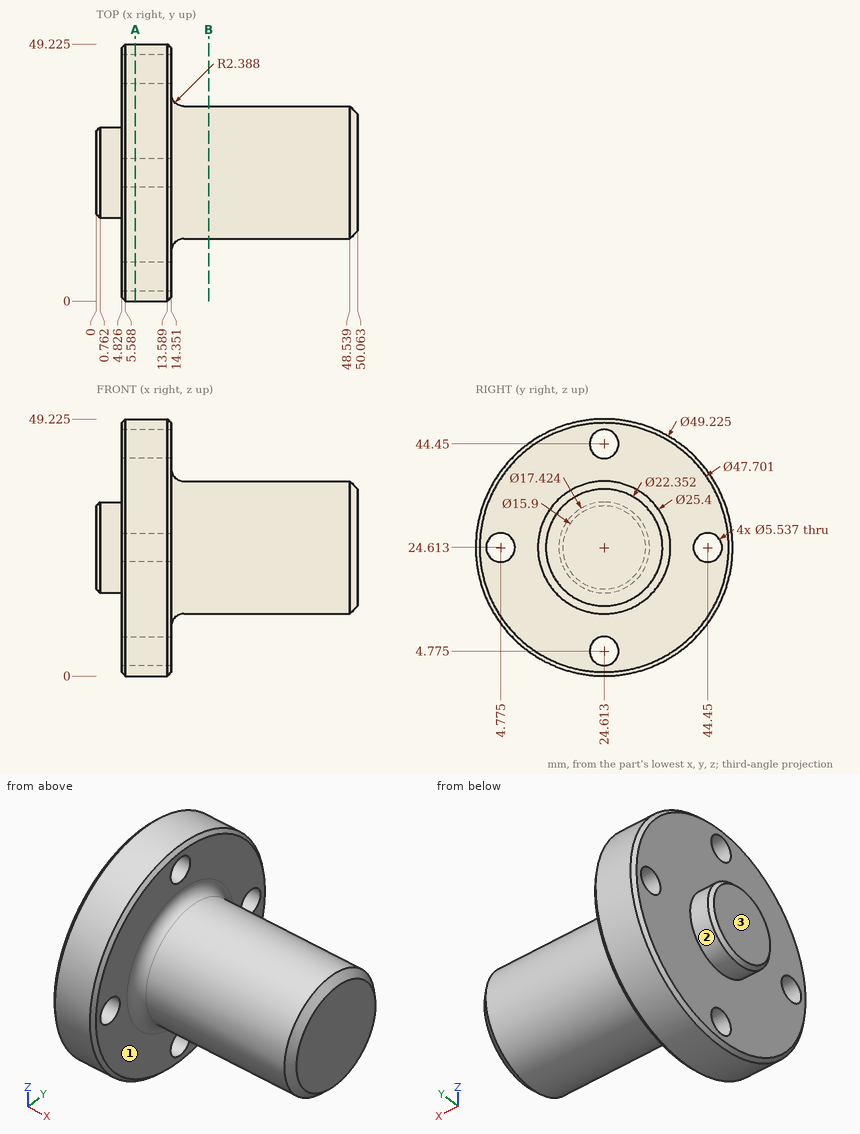
For this review, use the dimensioned drawing (mm, ordinates from the lowest corner) and the shaded views. A direction names the side the tool comes from. Give positions to 0.01 mm unless a question says otherwise; leave off trailing zeros. Order: outer loops, then holes, each group sorted by start corner. A loop starts at its lowest first (then second) coordinate and runs counter-clockwise, first axis right, second up. Notation, with made-up numbers: (-30.5, 33) - (26.5, 33) arc R23 cw to (26.5, 52) - close; hole circle Ø9 at (65, 4.5). An arc over 180 degrees is marked (long way). Use CSV: the item, a comma, the result in double quotes. Start each with the question number.
Q1. We need section A-A, the plane x = 7.5. State how many separate pieces and enclosed holes the cut face has, and give its area (3 significant figures).
Q2. To check wall thickness, follow line 1 along X through (y, z) = (30, 34); line 2 along X through (y, z) = (9, 33); line 3 along Y through (x, z) = (7.5, 44.45) (1 decimal). State the ranges of each line that lie inside material, in increasing order. Write a range as [from, to].
Q3. Clearance check with flat-ended pins moving along their axes: pin 1 Ø9 at (y, z) = (44.45, 24.61) entering from -X; pin 2 Ø4 at (x, z) = (33.5, 34.5) entering from -Y; pin 3 Ø3 at (y, z) = (12.5, 38.5) entering from +X; pin 4 Ø3.5 at (y, z) = (24.61, 44.45) entering from -X. State where each tip first meets the part, or that it passes through.
Q4. Tool access review of the marked faces 1, 2 and 3: name each direction out of +Z, -Z, +X, -X, +Y, -Y from which nothing blocks a thin tool from reaching the whole face with its end or side.
Q5. We need section B-B, the plane x = 21.5. Write out the cut boundary in (y, z), and give its area (3 significant figures).
Outcome:
1,separate pieces,"1"
1,enclosed holes,"4"
1,area,"1,810 mm^2"
2,line 1,"x = [4.83, 50.06]"
2,line 2,"x = [4.83, 14.35]"
2,line 3,"y = [10, 21.8], [27.4, 39.2]"
3,pin 1,"stops at x = 4.83"
3,pin 2,"stops at y = 14.66"
3,pin 3,"stops at x = 14.35"
3,pin 4,"passes through"
4,face 1,"+X"
4,face 2,"-X"
4,face 3,"+Z, -Z, -X, +Y, -Y"
5,outline,"circle Ø25.4 at (24.61, 24.61)"
5,area,"507 mm^2"
